Work out the finished part from the listing and answer in its coordinate system (mm). Round coordinates to 2 decimals unless told otherwise and drop trailing zeros. Write each loop counter-clockwise with the first axis right and the second up, starting at its lowest first coordinate (ties: lowest second). Pieces come first, ordered by that corner, then holes.
1. Find section A-A (x = -5). Write down the section's boundary in (y, z).
2. Find section B-B (z = -0.5). Write down the section's boundary in (x, y) (3 decimals), and give its area (3 significant figures).
3. Straight lines are drawn through the part: probe 1 along X at (y, z) = (-0.8, 23.5) (3 decimals); probe 2 along Z at (x, y) = (18.5, -1.2); probe 3 along X at (y, z) = (-0.75, -10). For each, find the intervals that lie inside material, in ascending order.
4. Flat-ended cylindrical pins translate along their axes: pin 1 Ø1.1 at (x, y) = (45, -2.5) entering from +Z; pin 2 Ø12 at (x, z) = (0, 46) entering from +Y; pin 3 Ø1.9 at (x, y) = (44.5, -2.5) entering from -Z. Find the tip coordinate at first contact, or state that the pin passes through.
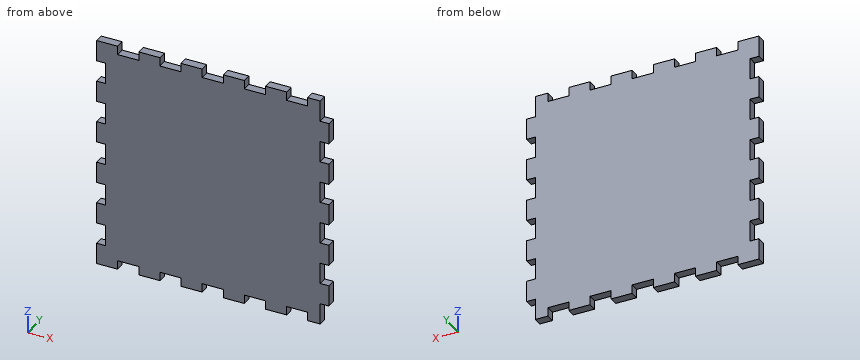
```python
from build123d import *

# Parameters (mm, degrees)
F1_DEPTH = 3.81


with BuildPart() as f1:
    # F0 (on Front) → F1 (new body)
    with BuildSketch(Plane.XZ):
        Polygon((-46.355, 61.0616), (-55.626, 61.0616), (-55.626, 51.7906), (-51.7906, 51.7906), (-51.7906, 42.5196), (-55.626, 42.5196), (-55.626, 33.2486), (-51.7906, 33.2486), (-51.7906, 23.9776), (-55.626, 23.9776), (-55.626, 14.7066), (-51.7906, 14.7066), (-51.7906, 5.4356), (-55.626, 5.4356), (-55.626, -3.8354), (-51.7906, -3.8354), (-51.7906, -13.1064), (-55.626, -13.1064), (-55.626, -22.3774), (-51.7906, -22.3774), (-51.7906, -31.6484), (-55.626, -31.6484), (-55.626, -40.9194), (-46.355, -40.9194), (-46.355, -37.084), (-37.084, -37.084), (-37.084, -40.9194), (-27.813, -40.9194), (-27.813, -37.084), (-18.542, -37.084), (-18.542, -40.9194), (-9.271, -40.9194), (-9.271, -37.084), (0, -37.084), (0, -40.9194), (9.271, -40.9194), (9.271, -37.084), (18.542, -37.084), (18.542, -40.9194), (27.813, -40.9194), (27.813, -37.084), (37.084, -37.084), (37.084, -40.9194), (42.545, -40.9194), (42.545, -31.6484), (46.3804, -31.6484), (46.3804, -22.3774), (42.545, -22.3774), (42.545, -13.1064), (46.3804, -13.1064), (46.3804, -3.8354), (42.545, -3.8354), (42.545, 5.4356), (46.3804, 5.4356), (46.3804, 14.7066), (42.545, 14.7066), (42.545, 23.9776), (46.3804, 23.9776), (46.3804, 33.2486), (42.545, 33.2486), (42.545, 42.5196), (46.3804, 42.5196), (46.3804, 51.7906), (42.545, 51.7906), (42.545, 61.0616), (37.084, 61.0616), (37.084, 57.2262), (27.813, 57.2262), (27.813, 61.0616), (18.542, 61.0616), (18.542, 57.2262), (9.271, 57.2262), (9.271, 61.0616), (0, 61.0616), (0, 57.2262), (-9.271, 57.2262), (-9.271, 61.0616), (-18.542, 61.0616), (-18.542, 57.2262), (-27.813, 57.2262), (-27.813, 61.0616), (-37.084, 61.0616), (-37.084, 57.2262), (-46.355, 57.2262), align=None)
    extrude(amount=F1_DEPTH)


solid = f1.part
```
Worked answers:
1. outline: (-3.81, -37.08) - (0, -37.08) - (0, 57.23) - (-3.81, 57.23) - close
2. outline: (-55.626, -3.81) - (42.545, -3.81) - (42.545, 0) - (-55.626, 0) - close
2. area: 374 mm2
3. probe 1: x = -55.626 to 42.545
3. probe 2: z = -37.08 to 57.23
3. probe 3: x = -51.79 to 46.38
4. pin 1: stops at z = 51.79
4. pin 2: stops at y = 0
4. pin 3: stops at z = -31.65
